from build123d import *

# Parameters (mm, degrees)
SKETCH1_R           = 25
SKETCH1_R_2         = 20
BOSS_EXTRUDE1_DEPTH = 10
BOSS_EXTRUDE2_DEPTH = 10
BOSS_EXTRUDE3_DEPTH = 10
FILLET1_R           = 10
SKETCH2_R           = 2
CUT_EXTRUDE1_DEPTH  = 10
CHAMFER1_SIZE       = 2
FILLET2_R           = 10
CHAMFER2_SIZE       = 2
FILLET3_R           = 1


with BuildPart() as part:
    # Sketch1 → Boss-Extrude1 (new body)
    with BuildSketch(Plane(origin=(0, 0, 0), x_dir=(1, 0, 0), z_dir=(0, 1, 0))):
        Circle(SKETCH1_R)
        Circle(SKETCH1_R_2, mode=Mode.SUBTRACT)
    extrude(amount=BOSS_EXTRUDE1_DEPTH)

    # Sketch3 → Boss-Extrude2 (add)
    with BuildSketch(Plane(origin=(0, 10, 0), x_dir=(1, 0, 0), z_dir=(0, 1, 0))):
        with BuildLine():
            Line((-25, -26), (25, -26))
            Line((25, -26), (25, 0))
            ThreePointArc((25, 0), (0, -25), (-25, 0))
            Line((-25, 0), (-25, -26))
        make_face()
    extrude(amount=-BOSS_EXTRUDE2_DEPTH)

    # Sketch4 → Boss-Extrude3 (add)
    with BuildSketch(Plane(origin=(0, 10, 0), x_dir=(1, 0, 0), z_dir=(0, 1, 0))):
        with BuildLine():
            Line((0, 35.355339059), (-17.67766953, 17.67766953))
            ThreePointArc((-17.67766953, 17.67766953), (0, 25), (17.67766953, 17.67766953))
            Line((17.67766953, 17.67766953), (0, 35.355339059))
        make_face()
    extrude(amount=-BOSS_EXTRUDE3_DEPTH)

    # Fillet1
    fillet1_edges = [part.edges().sort_by_distance(p)[0] for p in [
        (0, 5, -35.355339059),
    ]]
    fillet(fillet1_edges, radius=FILLET1_R)

    # Sketch2 → Cut-Extrude1 (cut)
    with BuildSketch(Plane(origin=(0, 10, 0), x_dir=(1, 0, 0), z_dir=(0, 1, 0))):
        with Locations((-21.335, -16)):
            Circle(SKETCH2_R)
        with Locations((0, 26.5)):
            Circle(SKETCH2_R)
        with Locations((21.335, -16)):
            Circle(SKETCH2_R)
    extrude(amount=-CUT_EXTRUDE1_DEPTH, mode=Mode.SUBTRACT)

    # Chamfer1
    chamfer1_edges = [part.edges().sort_by_distance(p)[0] for p in [
        (-20, 0, 0),
    ]]
    chamfer(chamfer1_edges, length=CHAMFER1_SIZE)

    # Fillet2
    fillet2_edges = [part.edges().sort_by_distance(p)[0] for p in [
        (-25, 5, 26),
        (25, 5, 26),
    ]]
    fillet(fillet2_edges, radius=FILLET2_R)

    # Chamfer2
    chamfer2_edges = [part.edges().sort_by_distance(p)[0] for p in [
        (-20, 10, 0),
    ]]
    chamfer(chamfer2_edges, length=CHAMFER2_SIZE)

    # Fillet3
    fillet3_edges = [part.edges().sort_by_distance(p)[0] for p in [
        (-25, 0, 8),
        (-25, 10, 8),
        (23.096988313, 0, -9.567085809),
        (-23.096988313, 0, -9.567085809),
        (-23.096988313, 10, -9.567085809),
        (-12.374368671, 10, -22.980970389),
        (-12.374368671, 0, -22.980970389),
        (12.374368671, 10, -22.980970389),
        (12.374368671, 0, -22.980970389),
        (0, 10, -31.213203436),
        (0, 0, -31.213203436),
        (23.096988313, 10, -9.567085809),
        (0, 10, 26),
        (0, 0, 26),
        (25, 10, 8),
        (-22.071067812, 10, 23.071067812),
        (22.071067812, 10, 23.071067812),
        (25, 0, 8),
        (-22.071067812, 0, 23.071067812),
        (22.071067812, 0, 23.071067812),
    ]]
    fillet(fillet3_edges, radius=FILLET3_R)


solid = part.part
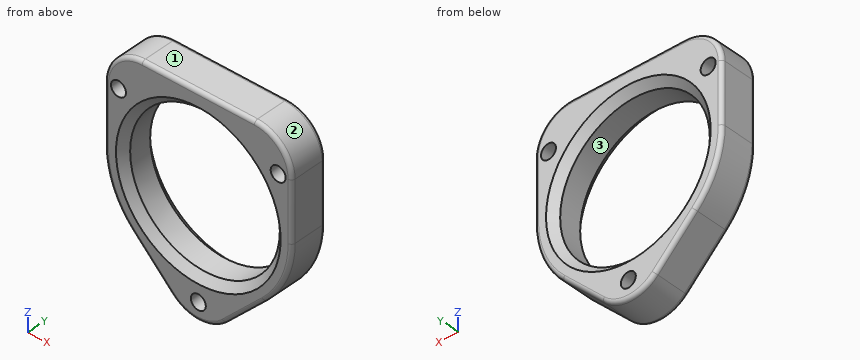
Work out the finished part from the listing and answer in its coordinate system (mm). Face numbers are marked on the shaded views. Round coordinates to 2 decimals unless told otherwise and drop trailing zeros. Loops run counter-clockwise (first coordinate to the right, second up) from the corner with the lowest first, then second, coordinate; pieces in that order, holes last. Notation, with made-up numbers: M -33,-22.5 L -10,-22.5 A36 cw -10,14.5 Z; hole C 2.5,-17 d8. An arc over 180 degrees is marked long. One line per question, with ' | ' between items. Start each with the question number.
(1) For a pull along X with two mould halves and no side action, classify the marked faces 1, 2 and 3 as released by +X, released by -X, zero draft, split by the parting line, or undercut.
(2) Find the intervals of material crossed by line 1 (Z direction, x = 0, y = 6.15); line 2 (Z direction, x = -0.5, y = 3.75); line 3 (X direction, y = 4, z = 16) (3 decimals), in increasing order.
(3) Flat-ended cylindrical pins translate along their axes: pin 1 Ø3 at (x, z) = (21.335, 16) entering from +Y; pin 2 Ø6 at (y, z) = (4, -12) entering from +X; pin 3 Ø6 at (y, z) = (6, -21) entering from +X; pin 4 Ø6 at (x, y) = (4, 5.5) entering from -Z. Find the tip coordinate at first contact, or state that the pin passes through.
(4) A cutting plane is placed at C-C on z = 15. Give the number of separate pieces and of enclosed holes in the cut face, plus the area to 3 significant figures.
(5) A cutting plane is placed at B-B on y = 4. Write down the section's boundary in (x, z) (3 decimals).
(6) A cutting plane is placed at A-A on x = 0. Write down the section's boundary in (y, z).
Geometry check:
1) face 1: zero draft | face 2: released by +X | face 3: undercut
2) line 1: z = -31.21 to -28.5, -24.5 to -20, 20 to 26 | line 2: z = -31.2 to -28.44, -24.56 to -19.99, 19.99 to 26 | line 3: x = -25 to -23.335, -19.335 to -12, 12 to 19.335, 23.335 to 25
3) pin 1: passes through | pin 2: stops at x = 23.32 | pin 3: stops at x = 17.36 | pin 4: stops at z = -31.16
4) separate pieces: 4 | enclosed holes: 0 | area: 154 mm²
5) outline: M -25,0 A25 ccw -17.678,-17.678 L -7.071,-28.284 A10 ccw 7.071,-28.284 L 17.678,-17.678 A25 ccw 25,0 L 25,16 A10 ccw 15,26 L -15,26 A10 ccw -25,16 Z; hole C -21.335,16 d4; hole C 0,0 d40; hole C 0,-26.5 d4; hole C 21.335,16 d4
6) outline: M 0,-30.21 A1 ccw 1,-31.21 L 9,-31.21 A1 ccw 10,-30.21 L 10,-28.5 L 0,-28.5 Z; M 0,-24.5 L 10,-24.5 L 10,-22 L 8,-20 L 2,-20 L 0,-22 Z; M 0,22 L 2,20 L 8,20 L 10,22 L 10,25 A1 ccw 9,26 L 1,26 A1 ccw 0,25 Z
